The figure shows three views and two pictorial views of one solid part (mm, origin at its lowest corner). Answer the questions. A direction names the side the tool comes from. Give positions to 0.01 mm unless a question says otherwise; leave off trailing zeros. Loops run counter-clockwise (first coordinate to the right, second up) from the corner with the lowest first, then second, coordinate; pieces in that order, holes last. Notation, with made-up numbers: M 43.25,-3.5 L 47.25,-3.5 A20 ccw 47.25,7.5 Z; hole C -3,58 d3. An arc over 180 degrees is marked long. Write item = value, one per line. Start each with the question number.
1. Section A-A on z = 22.5 is taken. Determine the outline of the cut face in (x, y), plus the area to 3 significant figures.
2. Section B-B on x = 7.5 is taken. Determine the outline of the cut face in (y, z), plus the area to 3 significant figures.
3. Section C-C on y = 15.75 is taken. Determine the outline of the cut face in (x, z).
4. For the marked faces 1 and 2, determine the directions among +Z, -Z, +X, -X, +Y, -Y from which every point of the face is accessible in a straight line to the end or side of a thin tool.
5. Section D-D on z = 9.25 is taken. Determine the outline of the cut face in (x, y).
6. Flat-ended cylindrical pins translate along their axes: pin 1 Ø7.5 at (x, z) = (10, 16) entering from -Y; pin 2 Ø7 at (x, z) = (7.5, 22.5) entering from +Y; pin 3 Ø6 at (y, z) = (7, 13.5) entering from +X; pin 4 Ø1 at (x, y) = (7, 11.5) entering from +Z. Find the tip coordinate at first contact, or state that the pin passes through.
7. Consider L1, parallel to Y at x = 7.5, z = 1; L2, parallel to Z at x = 7.5, y = 59.9; L3, parallel to Y at x = 12.5, z = 20.5. Determine where each line is inside the solid, lowest interval first. Write a range as [from, to].
8. The mould has two halves that part along Y. Classify the marked faces 3, 4 and 5: released by +Y, released by -Y, zero draft, split by the parting line, or undercut.
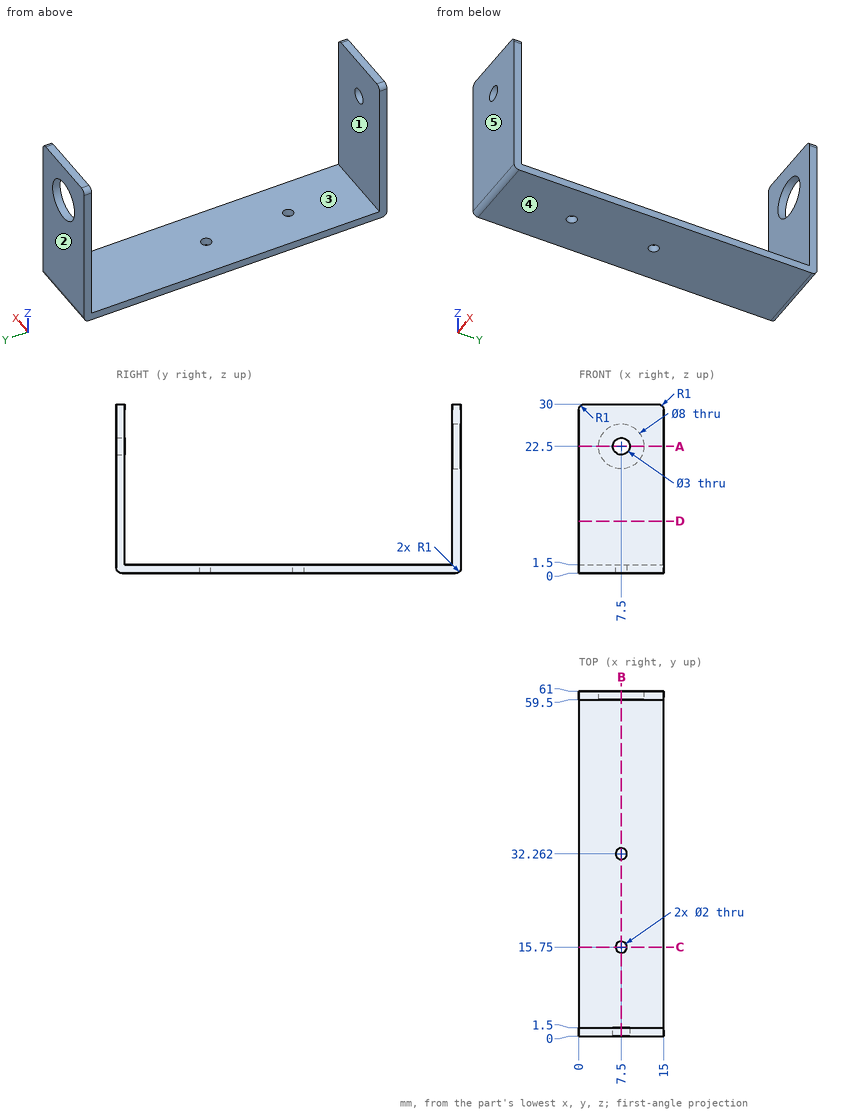
Verdict:
q1.outline = M 0,0 L 6,0 L 6,1.5 L 0,1.5 Z; M 0,59.5 L 3.5,59.5 L 3.5,61 L 0,61 Z; M 9,0 L 15,0 L 15,1.5 L 9,1.5 Z; M 11.5,59.5 L 15,59.5 L 15,61 L 11.5,61 Z
q1.area = 28.5 mm2
q2.outline = M 0,1 A1 ccw 1,0 L 14.75,0 L 14.75,1.5 L 1.5,1.5 L 1.5,21 L 0,21 Z; M 0,24 L 1.5,24 L 1.5,30 L 0,30 Z; M 16.75,0 L 31.26,0 L 31.26,1.5 L 16.75,1.5 Z; M 33.26,0 L 60,0 A1 ccw 61,1 L 61,18.5 L 59.5,18.5 L 59.5,1.5 L 33.26,1.5 Z; M 59.5,26.5 L 61,26.5 L 61,30 L 59.5,30 Z
q2.area = 154 mm2
q3.outline = M 0,0 L 6.5,0 L 6.5,1.5 L 0,1.5 Z; M 8.5,0 L 15,0 L 15,1.5 L 8.5,1.5 Z
q4.face_1 = +Z, +X, -X
q4.face_2 = +Z, -Z, +X, -X, +Y
q5.outline = M 0,0 L 15,0 L 15,1.5 L 0,1.5 Z; M 0,59.5 L 15,59.5 L 15,61 L 0,61 Z
q6.pin_1 = 0
q6.pin_2 = 1.5
q6.pin_3 = through
q6.pin_4 = 1.5
q7.L1 = [0, 14.75], [16.75, 31.26], [33.26, 61]
q7.L2 = [0, 18.5], [26.5, 30]
q7.L3 = [0, 1.5], [59.5, 61]
q8.face_3 = undercut
q8.face_4 = zero draft
q8.face_5 = released by -Y
